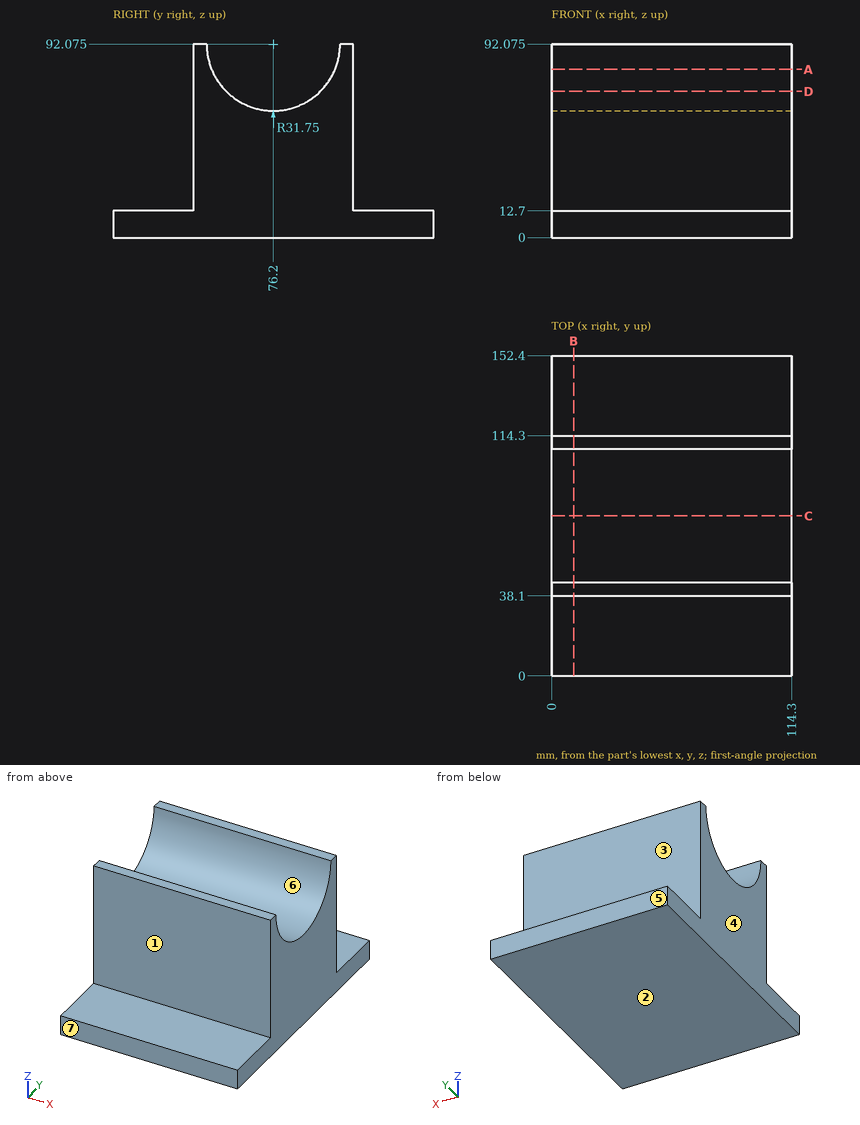
Verification items for this drawing (mm, ordinates from the low corner). A direction names the side the tool comes from. Round coordinates to 2 decimals unless told otherwise and drop trailing zeros. Loops run counter-clockwise (first coordinate to the right, second up) from the corner with the lowest first, then second, coordinate; pieces in that order, holes last. Notation, with made-up numbers: (-15, 44.5) -> (36, 44.5) arc R30 ccw to (36, 68.5) -> close; hole circle Ø7 at (-10, 29). An arc over 180 degrees is marked (long way). Write item = value, one per line. Start each with the question number.
1) Set-up check for the marked faces 1, 2 and 3: record each of +Z, -Z, +X, -X, +Y, -Y from which the full face is reachable in a straight line by a thin tool's end or side.
2) Sectioned sample at D-D, the plane z = 69.5. Record the cut outline in (x, y).
3) Release check for a two-part mould opening along Y. For the marked faces 4, 5, 6 and 7 record: released by +Y, released by -Y, zero draft, split by the parting line, or undercut.
4) Thickness scan on probe 1 along Y at (x, z) = (16, 57); probe 2 along Z at (x, y) = (104, 126.5); probe 3 along Y at (x, z) = (73, 83.5). Record the ranges inside material, lowest first.
5) Gauge pin test, flat ends, axial feed: pin 1 Ø19 at (x, y) = (84.5, 136.5) entering from +Z; pin 2 Ø6 at (x, y) = (101.5, 59.5) entering from -Z; pin 3 Ø10 at (x, z) = (47.5, 42.5) entering from -Y; pin 4 Ø4 at (x, z) = (51.5, 57.5) entering from +Y. Record the tip position at first contact, or that the pin passes through.
6) Sectioned sample at B-B, the plane x = 10.5. Record the cut outline in (y, z) (3 decimals).
7) Sectioned sample at C-C, the plane y = 76.2. Record the cut outline in (x, z) (3 decimals), plus the area to 3 significant figures.
8) Sectioned sample at A-A, the plane z = 80. Record the cut outline in (x, y), plus the area to 3 significant figures.
Results are:
q1.face_1 = +Z, +X, -X, -Y
q1.face_2 = -Z, +X, -X, +Y, -Y
q1.face_3 = +Z, +X, -X, +Y
q2.outline = (0, 38.1) -> (114.3, 38.1) -> (114.3, 53.87) -> (0, 53.87) -> close; (0, 98.53) -> (114.3, 98.53) -> (114.3, 114.3) -> (0, 114.3) -> close
q3.face_4 = zero draft
q3.face_5 = released by +Y
q3.face_6 = undercut
q3.face_7 = released by -Y
q4.probe_1 = 38.1 to 114.3
q4.probe_2 = 0 to 12.7
q4.probe_3 = 38.1 to 45.63, 106.77 to 114.3
q5.pin_1 = 12.7
q5.pin_2 = 0
q5.pin_3 = 38.1
q5.pin_4 = 114.3
q6.outline = (0, 0) -> (152.4, 0) -> (152.4, 12.7) -> (114.3, 12.7) -> (114.3, 92.075) -> (107.95, 92.075) arc R31.75 cw to (44.45, 92.075) -> (38.1, 92.075) -> (38.1, 12.7) -> (0, 12.7) -> close
q7.outline = (0, 0) -> (114.3, 0) -> (114.3, 60.325) -> (0, 60.325) -> close
q7.area = 6,900 mm^2
q8.outline = (0, 38.1) -> (114.3, 38.1) -> (114.3, 46.84) -> (0, 46.84) -> close; (0, 105.56) -> (114.3, 105.56) -> (114.3, 114.3) -> (0, 114.3) -> close
q8.area = 2,000 mm^2
